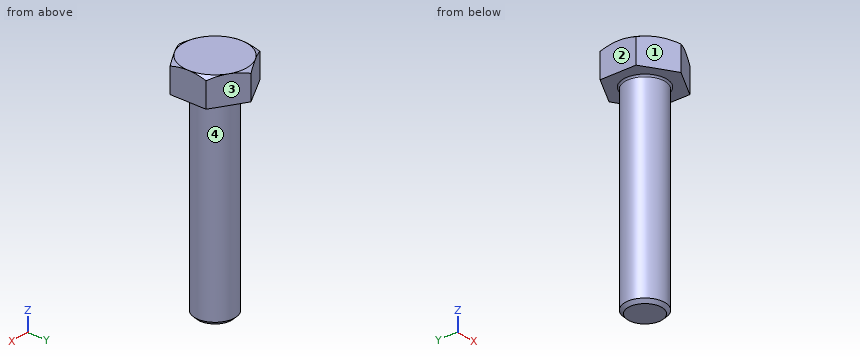
Autodesk Inventor part; units mm, degrees
ref_plane "WorkPlane1" through (0, 0, 0) normal (0, 0, 1) x (1, 0, 0)
ref_plane "MSC_PF1" through (0, 0, 0) normal (1, 0, 0) x (0, 1, 0)
ref_plane "MSC_PT1" through (0, 0, 0) normal (0, 0, -1) x (-1, 0, 0)
ref_plane "WorkPlane1" through (0, 0, 0) normal (0, 0, 1) x (1, 0, 0)
sketch "Sketch1" plane through (0, 0, 0) normal (0, 0, 1) x (1, 0, 0)
  point P0 (0, 0)
sketch "Sketch2" plane through (0, 0, 0) normal (0, 0, 1) x (1, 0, 0)
  line L0 (-4, 2.3095) -> (-4, -2.3095)
  line L1 (0, 4.6187) -> (-4, 2.3095)
  line L2 (4, 2.3095) -> (0, 4.6187)
  line L3 (4, -2.3095) -> (4, 2.3095)
  line L4 (0, -4.6187) -> (4, -2.3095)
  line L5 (-4, -2.3095) -> (0, -4.6187)
  circle A0 centre (0, 0) radius 4 construction
  dimension "d1" = 8
  dimension "d29" = 0
  dimension "d30" = 0
extrude "Extrusion1" add sketch "Sketch2" along normal blind 3.5
sketch "Sketch3" plane through (0, 0, 0) normal (1, 0, 0) x (0, 1, 0)
  line L0 (4, 3.5) -> (4.7187, 3.5)
  line L1 (4.7187, 3.085) -> (4, 3.5)
  line L2 (4.7187, 3.5) -> (4.7187, 3.085)
  line L3 (0, -0.7) -> (0, 4.2)
  line L4 (4.6187, 0) -> (4.6187, 3.5)
  dimension "d25" = 0.1
  dimension "d26" = 0
  dimension "d27" = 60
  dimension "d28" = 4
revolve "Revolution1" cut sketch "Sketch3" angle 360 about axis through (0, 0, -10) along (0, 0, 1)
sketch "Sketch4" plane through (0, 0, 0) normal (1, 0, 0) x (0, 1, 0)
  line L0 (0, -25) -> (0, 0)
  line L1 (-2.5, -25) -> (0, -25)
  line L2 (-2.5, 0) -> (-2.5, -25)
  line L3 (0, 0) -> (-2.5, 0)
  line L4 (0, -25) -> (0, 0)
  line L5 (-3, 0) -> (0.5, 0)
  line L6 (0, -30) -> (0, 5)
  dimension "d18" = 2.5
  dimension "d20" = 25
  dimension "d33" = 0
  dimension "d34" = 0
revolve "Revolution2" add sketch "Sketch4" angle 360 about axis through (0, 0, -25) along (0, 0, -1)
chamfer "Chamfer1" distance 0.4 angle 45 1 edges at (0, 2.5, -25)
fillet "Fillet1" radius 0.2 1 edges at (0, 2.5, 0)
thread "Thread1"
ref_plane "MSC_PF1" through (0, 0, 0) normal (1, 0, 0) x (0, 1, 0)
ref_plane "MSC_PT1" through (0, 0, 0) normal (0, 0, -1) x (-1, 0, 0)
equation "\"d22\" = 0.5 * PTC"
equation "\"d23\" = 0.5 * PTC"
equation "\"d24\" = r"
equation "\"d1\" = ParS"
equation "\"d6\" = ParK"
equation "\"d28\" = 0.5 * ParS"
equation "\"d18\" = 0.5 * NND"
equation "\"d20\" = NLG"
equation "\"NND\" = 5"
equation "\"NLG\" = 25"
equation "\"PTC\" = 0.8"
equation "\"ParK\" = 3.5"
equation "\"ParS\" = 8"
equation "\"msp_es\" = 0.577367 * ParS"
equation "\"r\" = 0.2"
equation "\"THREADDIA\" = NND"
properties part number "ISO 4016 - M5 x 25" material "Steel"
CAD build for the part. Positions are in the model's coordinates, mm. Face numbers are marked on the shaded views. Give positions to 0.01 mm unless a question says otherwise; leave off trailing zeros. Loops run counter-clockwise (first coordinate to the right, second up) from the corner with the lowest first, then second, coordinate; pieces in that order, holes last. Notation, with made-up numbers: M 88.25,18 L 118.25,18 A25 ccw 118.25,53 Z; hole C -32.5,-31.5 d6. An arc over 180 degrees is marked long. One line per question, with ' | ' between items. Start each with the question number.
1. Probe L1, parallel to Y at x = 0, z = -10.25; L2, parallel to Z at x = -3.25, y = 0.25. List the from-to ranges inside material, lowest first. Write a range as from..to.
2. Saw through at A-A on z = -13.75. Give the cut face in (x, y).
3. Flat gauge pins, fed straight in: pin 1 (2 mm diameter, centred on x = 2.5, y = 2, fed in from -Z); pin 2 (4 mm diameter, centred on x = -1, z = -10, fed in from -Y); pin 3 (1.5 mm diameter, centred on x = 2, z = -2.5, fed in from +Y). Where does each tip first touch, or does it go through?
4. Two-plate mould, pull along Y, no slides. Class the marked faces 1, 2, 3 and 4: pulls with the +Y half, pulls with the -Y half, needs draft (parallel to the pull), parting line crosses it, or undercut.
Result sheet:
1) L1: y = -2.5..2.5 | L2: z = 0..3.5
2) outline: C 0,0 d5
3) pin 1: stops at z = -24.9 | pin 2: stops at y = -2.5 | pin 3: stops at y = 2.17
4) face 1: pulls with the -Y half | face 2: needs draft | face 3: pulls with the +Y half | face 4: parting line crosses it
